Read the model definition and answer for the solid it produces. Units are mm, in the model's axes. Coordinates: 2 decimals unless noted, no trailing zeros. Write each loop counter-clockwise with the first axis right and the second up, starting at its lowest first coordinate (ties: lowest second). Pieces come first, ordered by that corner, then holes.
Item 1: Straight lines are drawn through the part: probe 1 along X at (y, z) = (7.25, 0.4); probe 2 along Y at (x, z) = (3.5, 0.5); probe 3 along Y at (x, z) = (3.5, 1.1). For each, find the intervals that lie inside material, in ascending order.
Item 2: Section B-B (x = 51) is taken. Give the vertices of the cut face in (y, z), then the cut area to 3 significant figures.
Item 3: Section A-A (y = 6.25) is taken. Give the vertices of the cut face in (x, z), then the cut area to 3 significant figures.
Item 4: Each of these flat-tipped pins is pushed along its axis until it touches: P1, Ø0.8, axis at x = 40, z = 1, coming from the +Y side (3 decimals); P2, Ø0.8, axis at x = 73, z = 0.5, coming from the -Y side; P3, Ø3, axis at x = 3.5, y = 3.5, coming from the +Z side. Where does it stop, or does it pass through?
from build123d import *

# Parameters (mm, degrees)
SKETCH_R  = 1.75
PAD_DEPTH = 1.5
FILLET_R  = 1


with BuildPart() as part:
    # Sketch → Pad (new body)
    with BuildSketch(Plane.XY):
        with BuildLine():
            ThreePointArc((0, 3.5), (3.5, 0), (7, 3.5))
            Line((7, 3.5), (7, 10.5))
            ThreePointArc((10.5, 14), (8.025126, 12.974874), (7, 10.5))
            Line((10.5, 14), (63.5, 14))
            ThreePointArc((67, 10.5), (65.974874, 12.974874), (63.5, 14))
            Line((67, 3.5), (67, 10.5))
            ThreePointArc((67, 3.5), (70.5, 0), (74, 3.5))
            Line((74, 3.5), (74, 10.5))
            ThreePointArc((77.5, 14), (75.025126, 12.974874), (74, 10.5))
            ThreePointArc((77.5, 14), (81, 17.5), (77.5, 21))
            Line((3.5, 21), (77.5, 21))
            ThreePointArc((3.5, 21), (1.025126, 19.974874), (0, 17.5))
            Line((0, 3.5), (0, 17.5))
        make_face()
        with Locations((3.5, 3.5)):
            Circle(SKETCH_R, mode=Mode.SUBTRACT)
        with Locations((70.5, 3.5)):
            Circle(SKETCH_R, mode=Mode.SUBTRACT)
        with BuildLine():
            ThreePointArc((5.5, 18.25), (4.75, 17.5), (5.5, 16.75))
            Line((5.5, 16.75), (9.5, 16.75))
            ThreePointArc((9.5, 16.75), (10.25, 17.5), (9.5, 18.25))
            Line((9.5, 18.25), (5.5, 18.25))
        make_face(mode=Mode.SUBTRACT)
        with BuildLine():
            ThreePointArc((38.5, 18.25), (37.75, 17.5), (38.5, 16.75))
            Line((38.5, 16.75), (42.5, 16.75))
            ThreePointArc((42.5, 16.75), (43.25, 17.5), (42.5, 18.25))
            Line((42.5, 18.25), (38.5, 18.25))
        make_face(mode=Mode.SUBTRACT)
        with BuildLine():
            ThreePointArc((71.5, 18.25), (70.75, 17.5), (71.5, 16.75))
            Line((71.5, 16.75), (75.5, 16.75))
            ThreePointArc((75.5, 16.75), (76.25, 17.5), (75.5, 18.25))
            Line((75.5, 18.25), (71.5, 18.25))
        make_face(mode=Mode.SUBTRACT)
    extrude(amount=PAD_DEPTH)

    # Fillet
    fillet_edges = [part.edges().sort_by_distance(p)[0] for p in [
        (3.5, 0, 1.5),
    ]]
    fillet(fillet_edges, radius=FILLET_R)


solid = part.part
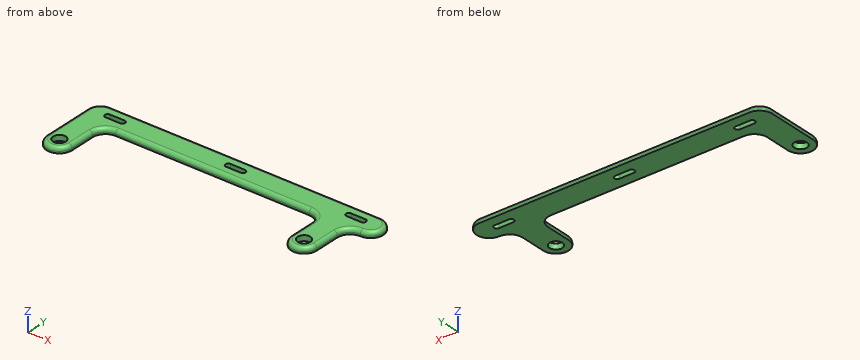
Established:
1. probe 1: x = 0 to 7, 67 to 74
1. probe 2: y = 0 to 1.75, 5.25 to 21
1. probe 3: y = 0.2 to 1.75, 5.25 to 20.8
2. outline: (14, 0) - (21, 0) - (21, 0.5) arc R1 ccw to (20, 1.5) - (15, 1.5) arc R1 ccw to (14, 0.5) - close
2. area: 10.1 mm2
3. outline: (0, 0) - (7, 0) - (7, 0.5) arc R1 ccw to (6, 1.5) - (1, 1.5) arc R1 ccw to (0, 0.5) - close; (67, 0) - (74, 0) - (74, 0.5) arc R1 ccw to (73, 1.5) - (68, 1.5) arc R1 ccw to (67, 0.5) - close
3. area: 20.1 mm2
4. P1: stops at y = 20.995
4. P2: stops at y = 0.7
4. P3: passes through
